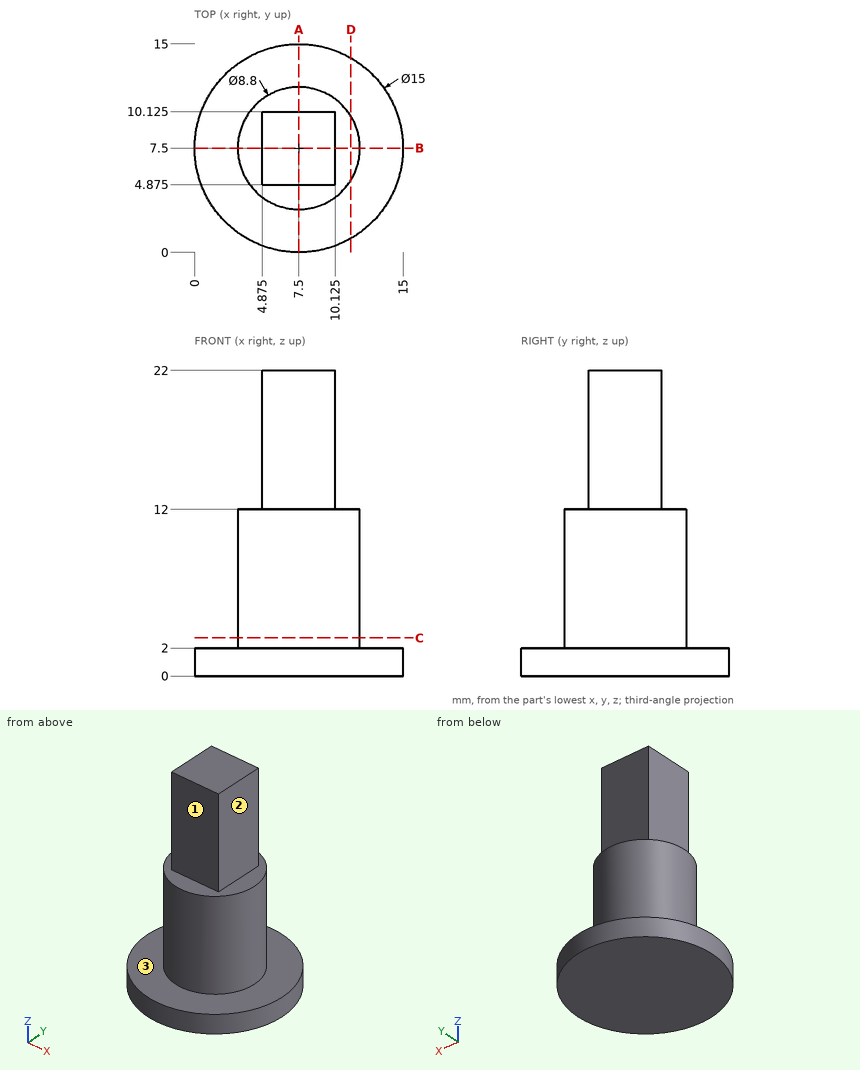
Design review of the part shown in the three views and the two pictorial views. Dimensions are in mm from the part's minimum x, y and z. A direction names the side the tool comes from. Round coordinates to 2 decimals unless told otherwise and drop trailing zeros. Loops run counter-clockwise (first coordinate to the right, second up) from the corner with the lowest first, then second, coordinate; pieces in that order, holes last.
1) Consider section A-A on x = 7.5. State the section outline as (y, z) points (3 decimals).
Values follow:
outline: (0, 0) - (15, 0) - (15, 2) - (11.9, 2) - (11.9, 12) - (10.125, 12) - (10.125, 22) - (4.875, 22) - (4.875, 12) - (3.1, 12) - (3.1, 2) - (0, 2) - close
2) Wall thickness on line 1 along Z through (x, y) = (1.75, 10); line 2 along Z through (x, y) = (10.5, 4.5); line 3 along Y through (x, z) = (8.25, 18) (3 decimals): over which ranges is each line inside the solid? List them lowest first.
Values follow:
line 1: z = 0 to 2
line 2: z = 0 to 12
line 3: y = 4.875 to 10.125
3) Tool access review of the marked faces 1, 2 and 3: name each direction out of +Z, -Z, +X, -X, +Y, -Y from which nothing blocks a thin tool from reaching the whole face with its end or side.
Values follow:
face 1: +Z, +X, -X, -Y
face 2: +Z, +X, +Y, -Y
face 3: +Z
4) Consider section D-D on x = 11.25. State the section outline as (y, z) points.
Values follow:
outline: (1, 0) - (14, 0) - (14, 2) - (9.8, 2) - (9.8, 12) - (5.2, 12) - (5.2, 2) - (1, 2) - close
5) Clearance check with flat-ended pins moving along their axes: P1, Ø1.5, axis at x = 4.5, y = 3, coming from the +Z side; P2, Ø1.6, axis at x = 7.5, z = 19, coming from the +Y side (3 decimals); P3, Ø1.6, axis at x = 6.5, z = 17, coming from the -Y side (3 decimals); P4, Ø2, axis at y = 2, z = 8, coming from the +X side. State where each tip first meets the part, or that it passes through.
Values follow:
P1: stops at z = 2
P2: stops at y = 10.125
P3: stops at y = 4.875
P4: passes through
6) Consider section C-C on z = 2.75. State the section outline as (x, y) points, then the cut area to 3 significant figures.
Values follow:
outline: circle Ø8.8 at (7.5, 7.5)
area: 60.8 mm2
